from build123d import *

# Parameters (mm, degrees)
F2_DEPTH = 25.4
F3_R     = 5.08
F4_R     = 5.08


with BuildPart() as f2:
    # F1 (on offset) → F2 (new body)
    with BuildSketch(Plane.YZ.offset(152.4)):
        Polygon((-28.573824, 50.16654), (-59.09586, 30.684389), (-58.771159, 0), (0.524219, 0.627459), (0, 50.16654), align=None)
    extrude(amount=F2_DEPTH)

    # F3
    f3_edges = [f2.edges().sort_by_distance(p)[0] for p in [
        (165.1, -58.771159, 0),
    ]]
    fillet(f3_edges, radius=F3_R)

    # F4
    f4_edges = [f2.edges().sort_by_distance(p)[0] for p in [
        (165.1, 0.524219, 0.627459),
        (165.1, 0, 50.16654),
    ]]
    fillet(f4_edges, radius=F4_R)


solid = f2.part
Could you check a few things on this model? Use its own coordinates, in mm. Give positions to 0.01 mm unless a question says otherwise; leave off trailing zeros. Order: outer loops, then holes, each group sorted by start corner. A loop starts at its lowest first (then second) coordinate and runs counter-clockwise, first axis right, second up. Notation, with made-up numbers: (60, 11) -> (108, 11) arc R31 cw to (108, 50) -> close; hole circle Ø9 at (-2, -36). An arc over 180 degrees is marked (long way). Answer in a Markdown table with one row per item. Add a question column.
Item 1: I'm going to push flat-ended pins straight in: P1, Ø3, axis at x = 169, z = 25, coming from the -Y side; P2, Ø4, axis at x = 174, z = 33.5, coming from the -Y side; P3, Ø1, axis at x = 168.5, z = 30.5, coming from the +Y side. Where does each tip first touch, or does it pass through?
Item 2: Imagine slicing it at A-A (x = 158). List the corners of the cut face in (y, z) for me, and give its area (3 significant figures).
Item 3: Please list where these lines run through material, in increasing order: probe 1 along Z at (x, y) = (166.25, -13.5); probe 2 along Y at (x, z) = (168, 26.5); probe 3 along Z at (x, y) = (153.75, -53.5).
Item 4: Imagine slicing it at C-C (z = 38). List the corners of the cut face in (x, y) for me.
Item 5: Imagine slicing it at B-B (y = -42.5). List the corners of the cut face in (x, z) for me, and give its area (3 significant figures).
Result:
| question | item | result |
|---|---|---|
| 1 | P1 | y = -59.05 |
| 1 | P2 | y = -57.82 |
| 1 | P3 | y = 0.21 |
| 2 | outline | (-59.1, 30.68) -> (-58.82, 5.08) arc R5.08 ccw to (-53.69, 0.05) -> (-4.56, 0.57) arc R5.08 ccw to (0.47, 5.71) -> (0.05, 45.14) arc R5.08 ccw to (-5.03, 50.17) -> (-28.57, 50.17) -> close |
| 2 | area | 2,640 mm2 |
| 3 | probe 1 | 0.48 to 50.17 |
| 3 | probe 2 | -59.05 to 0.25 |
| 3 | probe 3 | 0.06 to 34.26 |
| 4 | outline | (152.4, -47.63) -> (177.8, -47.63) -> (177.8, 0.13) -> (152.4, 0.13) -> close |
| 5 | outline | (152.4, 0.17) -> (177.8, 0.17) -> (177.8, 41.28) -> (152.4, 41.28) -> close |
| 5 | area | 1,040 mm2 |
